Read the model definition and answer for the solid it produces. Units are mm, in the model's axes. Round coordinates to 2 decimals unless told otherwise and drop trailing zeros. Write each loop counter-clockwise with the first axis right and the second up, starting at its lowest first coordinate (ties: lowest second). Pieces come first, ordered by that corner, then holes. Notation, with made-up numbers: (12.25, -22.5) -> (50.25, -22.5) arc R22 cw to (50.25, 15.5) -> close; hole circle Ø2 at (-3.5, 67.25). An arc over 180 degrees is marked (long way). Return JSON: item names as keys, results as strings.
from build123d import *

# Parameters (mm, degrees)
SKETCH_W          = 520.7
SKETCH_H          = 584.2
PAD_DEPTH         = 3.175
CYLINDER_R        = 1.75
CYLINDER_DEPTH    = 3.175
CYLINDER001_R     = 1.75
CYLINDER001_DEPTH = 3.175
CYLINDER002_R     = 1.75
CYLINDER002_DEPTH = 3.175
CYLINDER003_R     = 1.75
CYLINDER003_DEPTH = 3.175
CYLINDER004_R     = 52.9996
CYLINDER004_DEPTH = 3.175
CYLINDER005_R     = 2.54
CYLINDER005_DEPTH = 3.175
CYLINDER006_R     = 2.54
CYLINDER006_DEPTH = 3.175
CYLINDER007_R     = 2.54
CYLINDER007_DEPTH = 3.175
CYLINDER008_R     = 2.54
CYLINDER008_DEPTH = 3.175
BOX_W             = 30
BOX_H             = 22
BOX_DEPTH         = 3.2
CYLINDER009_R     = 1.9
CYLINDER009_DEPTH = 3.2
CYLINDER010_R     = 1.9
CYLINDER010_DEPTH = 3.2
CYLINDER011_R     = 2.54
CYLINDER011_DEPTH = 3.175
CYLINDER012_R     = 2.54
CYLINDER012_DEPTH = 3.175
CYLINDER013_R     = 2.54
CYLINDER013_DEPTH = 3.175
CYLINDER014_R     = 2.54
CYLINDER014_DEPTH = 3.175


with BuildPart() as part:
    # Sketch → Pad (new body)
    with BuildSketch(Plane.XZ):
        Rectangle(SKETCH_W, SKETCH_H)
    extrude(amount=PAD_DEPTH)

    # Cylinder → Cylinder (cut)
    with BuildSketch(Plane(origin=(-179.64912, 0, -118.1989), x_dir=(1, 0, 0), z_dir=(0, -1, 0))):
        Circle(CYLINDER_R)
    extrude(amount=CYLINDER_DEPTH, mode=Mode.SUBTRACT)

    # Cylinder001 → Cylinder001 (cut)
    with BuildSketch(Plane(origin=(-57.14912, 0, -203.1989), x_dir=(1, 0, 0), z_dir=(0, -1, 0))):
        Circle(CYLINDER001_R)
    extrude(amount=CYLINDER001_DEPTH, mode=Mode.SUBTRACT)

    # Cylinder002 → Cylinder002 (cut)
    with BuildSketch(Plane(origin=(-130.64912, 0, -178.6989), x_dir=(1, 0, 0), z_dir=(0, -1, 0))):
        Circle(CYLINDER002_R)
    extrude(amount=CYLINDER002_DEPTH, mode=Mode.SUBTRACT)

    # Cylinder003 → Cylinder003 (cut)
    with BuildSketch(Plane(origin=(-130.64912, 0, -145.6989), x_dir=(1, 0, 0), z_dir=(0, -1, 0))):
        Circle(CYLINDER003_R)
    extrude(amount=CYLINDER003_DEPTH, mode=Mode.SUBTRACT)

    # Cylinder004 → Cylinder004 (cut)
    with BuildSketch(Plane(origin=(0.00086, 0, 171.8011), x_dir=(1, 0, 0), z_dir=(0, -1, 0))):
        Circle(CYLINDER004_R)
    extrude(amount=CYLINDER004_DEPTH, mode=Mode.SUBTRACT)

    # Cylinder005 → Cylinder005 (cut)
    with BuildSketch(Plane(origin=(-52.4984, 0, 224.30036), x_dir=(1, 0, 0), z_dir=(0, -1, 0))):
        Circle(CYLINDER005_R)
    extrude(amount=CYLINDER005_DEPTH, mode=Mode.SUBTRACT)

    # Cylinder006 → Cylinder006 (cut)
    with BuildSketch(Plane(origin=(52.50012, 0, 224.30036), x_dir=(1, 0, 0), z_dir=(0, -1, 0))):
        Circle(CYLINDER006_R)
    extrude(amount=CYLINDER006_DEPTH, mode=Mode.SUBTRACT)

    # Cylinder007 → Cylinder007 (cut)
    with BuildSketch(Plane(origin=(52.50012, 0, 119.30184), x_dir=(1, 0, 0), z_dir=(0, -1, 0))):
        Circle(CYLINDER007_R)
    extrude(amount=CYLINDER007_DEPTH, mode=Mode.SUBTRACT)

    # Cylinder008 → Cylinder008 (cut)
    with BuildSketch(Plane(origin=(-52.4984, 0, 119.30184), x_dir=(1, 0, 0), z_dir=(0, -1, 0))):
        Circle(CYLINDER008_R)
    extrude(amount=CYLINDER008_DEPTH, mode=Mode.SUBTRACT)

    # Box → Box (cut)
    with BuildSketch(Plane(origin=(-152.4984, 0.025, -277.69816), x_dir=(1, 0, 0), z_dir=(0, -1, 0))):
        with Locations((15, 11)):
            Rectangle(BOX_W, BOX_H)
    extrude(amount=BOX_DEPTH, mode=Mode.SUBTRACT)

    # Cylinder009 → Cylinder009 (cut)
    with BuildSketch(Plane(origin=(-157.4984, 0.025, -266.69816), x_dir=(1, 0, 0), z_dir=(0, -1, 0))):
        Circle(CYLINDER009_R)
    extrude(amount=CYLINDER009_DEPTH, mode=Mode.SUBTRACT)

    # Cylinder010 → Cylinder010 (cut)
    with BuildSketch(Plane(origin=(-117.4984, 0.025, -266.69816), x_dir=(1, 0, 0), z_dir=(0, -1, 0))):
        Circle(CYLINDER010_R)
    extrude(amount=CYLINDER010_DEPTH, mode=Mode.SUBTRACT)

    # Cylinder011 → Cylinder011 (cut)
    with BuildSketch(Plane(origin=(-234.95054, 0, -266.7007), x_dir=(1, 0, 0), z_dir=(0, -1, 0))):
        Circle(CYLINDER011_R)
    extrude(amount=CYLINDER011_DEPTH, mode=Mode.SUBTRACT)

    # Cylinder012 → Cylinder012 (cut)
    with BuildSketch(Plane(origin=(-234.95054, 0, 266.6993), x_dir=(1, 0, 0), z_dir=(0, -1, 0))):
        Circle(CYLINDER012_R)
    extrude(amount=CYLINDER012_DEPTH, mode=Mode.SUBTRACT)

    # Cylinder013 → Cylinder013 (cut)
    with BuildSketch(Plane(origin=(234.94946, 0, 266.6993), x_dir=(1, 0, 0), z_dir=(0, -1, 0))):
        Circle(CYLINDER013_R)
    extrude(amount=CYLINDER013_DEPTH, mode=Mode.SUBTRACT)

    # Cylinder014 → Cylinder014 (cut)
    with BuildSketch(Plane(origin=(234.94946, 0, -266.7007), x_dir=(1, 0, 0), z_dir=(0, -1, 0))):
        Circle(CYLINDER014_R)
    extrude(amount=CYLINDER014_DEPTH, mode=Mode.SUBTRACT)


solid = part.part
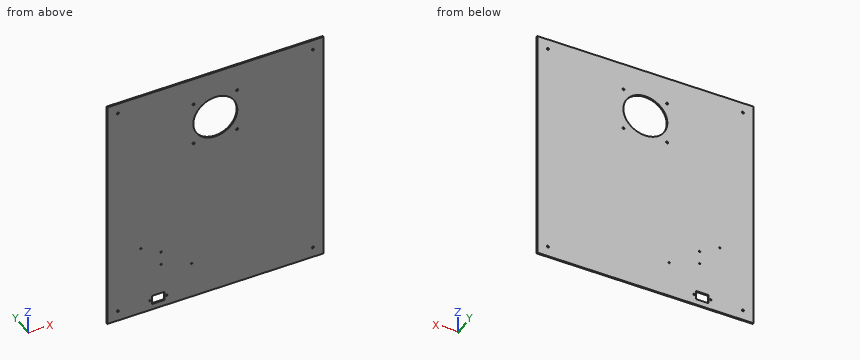
Item 1: Section C-C (x = -2) is taken. Give the vertices of the cut face in (y, z) (3 decimals), then the cut area to 3 significant figures.
Worked answers:
{"outline": "(-3.175, -292.1) -> (0, -292.1) -> (0, 118.839) -> (-3.175, 118.839) -> close; (-3.175, 224.763) -> (0, 224.763) -> (0, 292.1) -> (-3.175, 292.1) -> close", "area": "1,520 mm2"}
Item 2: Section A-A (z = 145) is taken. Give the vertices of the cut face in (x, y) (3 decimals).
Worked answers:
{"outline": "(-260.35, -3.175) -> (-45.723, -3.175) -> (-45.723, 0) -> (-260.35, 0) -> close; (45.725, -3.175) -> (260.35, -3.175) -> (260.35, 0) -> (45.725, 0) -> close"}
Item 3: Section B-B (y = -0.6) is taken. State how many separate pieces and enclosed holes the cut face has, then the cut area to 3 significant figures.
Worked answers:
{"separate pieces": "1", "enclosed holes": "16", "area": "294,000 mm2"}
Item 4: Straight lines are drawn through the part: L1, parallel to X at y = -2.75, z = 266; L2, parallel to X at y = -0.35, z = -146; L3, parallel to Z at x = 237, y = -2.65. For each, find the intervals that lie inside material, in ascending order. Write a range as [from, to].
Worked answers:
{"L1": "x = [-260.35, -237.39], [-232.51, 232.51], [237.39, 260.35]", "L2": "x = [-260.35, -132.37], [-128.93, 260.35]", "L3": "z = [-292.1, -268.2], [-265.2, 265.2], [268.2, 292.1]"}
